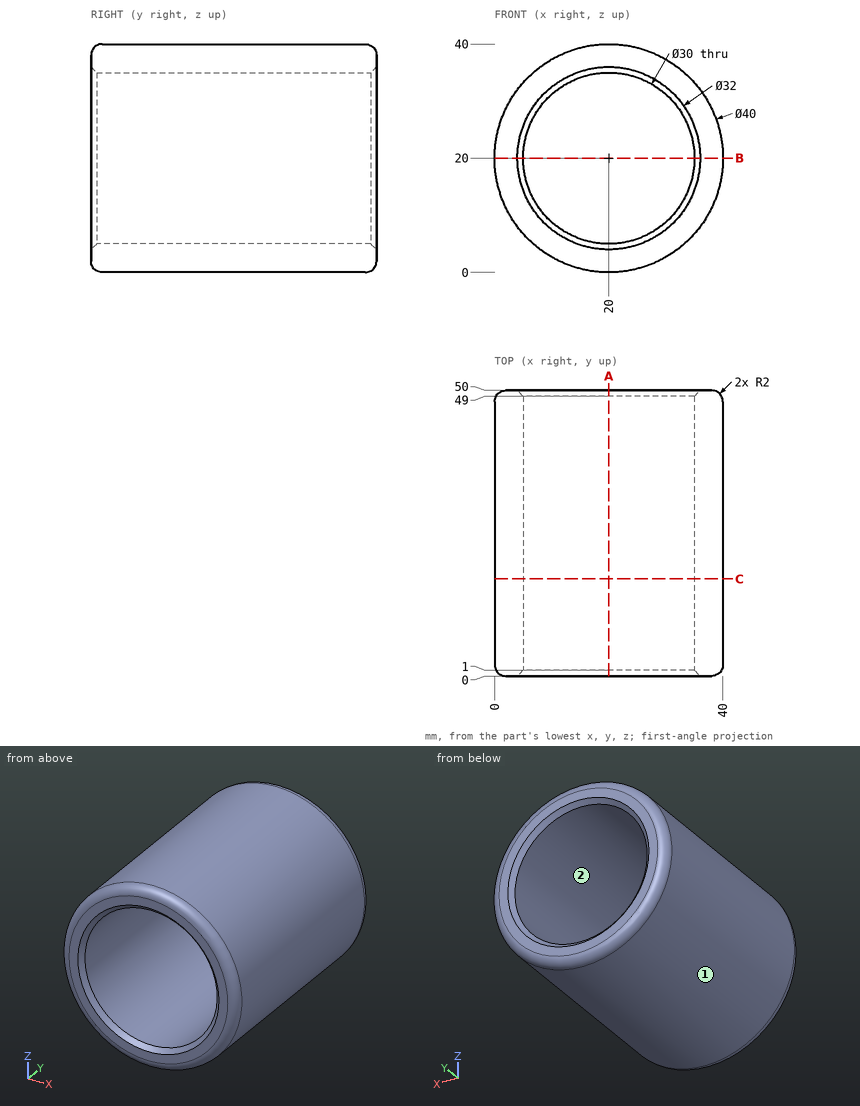
Design review of the part shown in the three views and the two pictorial views. Dimensions are in mm from the part's minimum x, y and z. Round coordinates to 2 decimals unless told otherwise and drop trailing zeros. Order: outer loops, then holes, each group sorted by start corner. A loop starts at its lowest first (then second) coordinate and runs counter-clockwise, first axis right, second up. Notation, with made-up numbers: (14.25, 25) -> (73.25, 25) arc R29 ccw to (73.25, 62) -> close; hole circle Ø11 at (-22, 38.5). An arc over 180 degrees is marked (long way). Write item = value, one per line. Start each with the question number.
1) Take a section at C-C on y = 17. State the section outline as (x, z) points, plus the area to 3 significant figures.
2) The part is to be moulded in two halves that separate along X. For the marked faces 1 and 2, say which applies: +X half, -X half, draft (parallel to the pull), parting line (faces both ways), or undercut.
3) Take a section at A-A on x = 20. State the section outline as (y, z) points.
4) Insertion check: pin 1 (24 mm diameter, centred on x = 20, z = 20, fed in from +Y); pin 2 (5 mm diameter, centred on x = 16.5, y = 7, fed in from +Z) (3 decimals); pin 3 (10 mm diameter, centred on x = 11, y = 38.5, fed in from +Z); pin 4 (6 mm diameter, centred on y = 21, z = 24.5, fed in from +X). Each pin has a flat end and moves straight along its axis. Give the tip position at first contact, or say it passes through.
5) To check wall thickness, follow line 1 (X direction, y = 14, z = 20); line 2 (Z direction, x = 26.5, y = 26); line 3 (X direction, y = 7, z = 18.5). State the ranges of each line that lie inside material, in increasing order. Write a range as from..to.
6) Take a section at B-B on z = 20. State the section outline as (x, y) points, plus the area to 3 significant figures.
Verdict:
q1.outline = circle Ø40 at (20, 20); hole circle Ø30 at (20, 20)
q1.area = 550 mm2
q2.face_1 = parting line
q2.face_2 = undercut
q3.outline = (0, 2) arc R2 ccw to (2, 0) -> (48, 0) arc R2 ccw to (50, 2) -> (50, 4) -> (49, 5) -> (1, 5) -> (0, 4) -> close; (0, 36) -> (1, 35) -> (49, 35) -> (50, 36) -> (50, 38) arc R2 ccw to (48, 40) -> (2, 40) arc R2 ccw to (0, 38) -> close
q4.pin_1 = through
q4.pin_2 = 39.975
q4.pin_3 = 39.6
q4.pin_4 = 39.94
q5.line_1 = 0..5, 35..40
q5.line_2 = 1.09..6.48, 33.52..38.91
q5.line_3 = 0.06..5.08, 34.92..39.94
q6.outline = (0, 2) arc R2 ccw to (2, 0) -> (4, 0) -> (5, 1) -> (5, 49) -> (4, 50) -> (2, 50) arc R2 ccw to (0, 48) -> close; (35, 1) -> (36, 0) -> (38, 0) arc R2 ccw to (40, 2) -> (40, 48) arc R2 ccw to (38, 50) -> (36, 50) -> (35, 49) -> close
q6.area = 495 mm2
